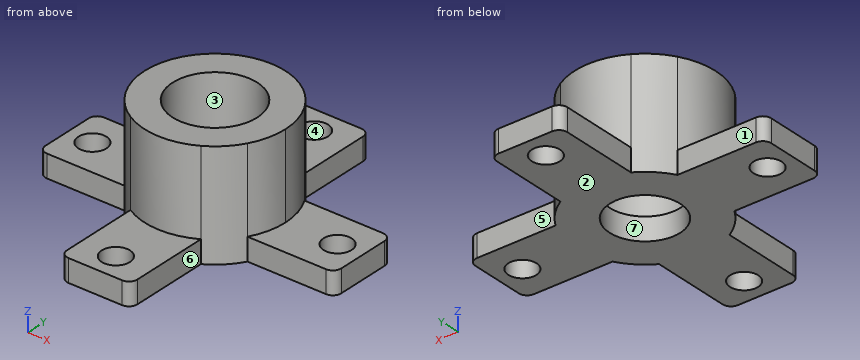
from build123d import *

# Parameters (mm, degrees)
F0_R     = 1
F0_W     = 5
F0_H     = 5
F1_DEPTH = 1.6
F2_R     = 3
F3_DEPTH = 6
F4_DEPTH = 1.6
F5_R     = 2.5
F6_DEPTH = 1.6


with BuildPart() as f1:
    # F0 (on Top) → F1 (new body)
    with BuildSketch(Plane.XY):
        with BuildLine():
            ThreePointArc((10.5, 1.9), (10.3242640687, 2.3242640687), (9.9, 2.5))
            Line((9.9, 2.5), (2.5, 2.5))
            Line((2.5, 2.5), (2.5, -2.5))
            Line((2.5, -2.5), (9.9, -2.5))
            ThreePointArc((9.9, -2.5), (10.3242640687, -2.3242640687), (10.5, -1.9))
            Line((10.5, -1.9), (10.5, 1.9))
        make_face()
        with Locations((8.7, 0)):
            Circle(F0_R, mode=Mode.SUBTRACT)
        Rectangle(F0_W, F0_H)
        with BuildLine():
            Line((-2.5, 2.5), (2.5, 2.5))
            Line((2.5, 2.5), (2.5, 9.9))
            ThreePointArc((2.5, 9.9), (2.3242640687, 10.3242640687), (1.9, 10.5))
            Line((1.9, 10.5), (-1.9, 10.5))
            ThreePointArc((-1.9, 10.5), (-2.3242640687, 10.3242640687), (-2.5, 9.9))
            Line((-2.5, 9.9), (-2.5, 2.5))
        make_face()
        with Locations((0, 8.7)):
            Circle(F0_R, mode=Mode.SUBTRACT)
        with BuildLine():
            Line((-2.5, -2.5), (-2.5, 2.5))
            Line((-2.5, 2.5), (-9.9, 2.5))
            ThreePointArc((-9.9, 2.5), (-10.3242640687, 2.3242640687), (-10.5, 1.9))
            Line((-10.5, 1.9), (-10.5, -1.9))
            ThreePointArc((-10.5, -1.9), (-10.3242640687, -2.3242640687), (-9.9, -2.5))
            Line((-9.9, -2.5), (-2.5, -2.5))
        make_face()
        with Locations((-8.7, 0)):
            Circle(F0_R, mode=Mode.SUBTRACT)
        with BuildLine():
            Line((2.5, -9.9), (2.5, -2.5))
            Line((2.5, -2.5), (-2.5, -2.5))
            Line((-2.5, -2.5), (-2.5, -9.9))
            ThreePointArc((-2.5, -9.9), (-2.3242640687, -10.3242640687), (-1.9, -10.5))
            Line((-1.9, -10.5), (1.9, -10.5))
            ThreePointArc((1.9, -10.5), (2.3242640687, -10.3242640687), (2.5, -9.9))
        make_face()
        with Locations((0, -8.7)):
            Circle(F0_R, mode=Mode.SUBTRACT)
    extrude(amount=F1_DEPTH)

    # F2 (on face) → F3 (join)
    with BuildSketch(Plane.XY.offset(1.6)):
        with BuildLine():
            ThreePointArc((4.3301270189, -2.5), (4.8296291314, -1.2940952255), (5, 0))
            ThreePointArc((5, 0), (4.8296291314, 1.2940952255), (4.3301270189, 2.5))
            Line((4.3301270189, 2.5), (2.5, 2.5))
            Line((2.5, 2.5), (2.5, 4.3301270189))
            ThreePointArc((2.5, 4.3301270189), (0, 5), (-2.5, 4.3301270189))
            Line((-2.5, 4.3301270189), (-2.5, 2.5))
            Line((-2.5, 2.5), (-4.3301270189, 2.5))
            ThreePointArc((-4.3301270189, 2.5), (-5, 0), (-4.3301270189, -2.5))
            Line((-4.3301270189, -2.5), (-2.5, -2.5))
            Line((-2.5, -2.5), (-2.5, -4.3301270189))
            ThreePointArc((-2.5, -4.3301270189), (0, -5), (2.5, -4.3301270189))
            Line((2.5, -4.3301270189), (2.5, -2.5))
            Line((2.5, -2.5), (4.3301270189, -2.5))
        make_face()
        Circle(F2_R, mode=Mode.SUBTRACT)
        with BuildLine():
            ThreePointArc((-4.3301270189, -2.5), (-3.5355339059, -3.5355339059), (-2.5, -4.3301270189))
            Line((-2.5, -4.3301270189), (-2.5, -2.5))
            Line((-2.5, -2.5), (-4.3301270189, -2.5))
        make_face()
        with BuildLine():
            ThreePointArc((2.5, -4.3301270189), (3.5355339059, -3.5355339059), (4.3301270189, -2.5))
            Line((4.3301270189, -2.5), (2.5, -2.5))
            Line((2.5, -2.5), (2.5, -4.3301270189))
        make_face()
        with BuildLine():
            Line((2.5, 2.5), (4.3301270189, 2.5))
            ThreePointArc((4.3301270189, 2.5), (3.5355339059, 3.5355339059), (2.5, 4.3301270189))
            Line((2.5, 4.3301270189), (2.5, 2.5))
        make_face()
        with BuildLine():
            Line((-2.5, 2.5), (-2.5, 4.3301270189))
            ThreePointArc((-2.5, 4.3301270189), (-3.5355339059, 3.5355339059), (-4.3301270189, 2.5))
            Line((-4.3301270189, 2.5), (-2.5, 2.5))
        make_face()
    extrude(amount=F3_DEPTH)

    # F4 (add, through all): faces of the model
    f4_faces = [f1.faces().sort_by_distance(p)[0] for p in [
        (-3.1629509292, 3.1629509292, 1.6),
        (3.1629509292, 3.1629509292, 1.6),
        (-3.1629509292, -3.1629509292, 1.6),
        (3.1629509292, -3.1629509292, 1.6),
    ]]
    extrude(f4_faces, amount=F4_DEPTH)

    # F5 (on face) → F6 (cut, through all)
    with BuildSketch(Plane.XY.offset(1.6)):
        Circle(F5_R)
    extrude(amount=-F6_DEPTH, mode=Mode.SUBTRACT)


solid = f1.part
Design review of the part built by this model. Coordinates are the model's own, in mm. Face numbers are marked on the shaded views. A direction names the side the tool comes from. Round coordinates to 2 decimals unless told otherwise and drop trailing zeros. Write each loop counter-clockwise with the first axis right and the second up, starting at its lowest first coordinate (ties: lowest second). Pieces come first, ordered by that corner, then holes. Notation, with made-up numbers: M 83,85.25 L 137,85.25 A17 ccw 137,105.25 Z; hole C -9,54 d11. An arc over 180 degrees is marked long. One line per item, written item: value. Start each with the question number.
1. Take a section at D-D on x = 5.5. State the section outline as (y, z) points, then the cut area to 3 significant figures.
2. Take a section at A-A on x = 0. State the section outline as (y, z) points, then the cut area to 3 significant figures.
3. Take a section at C-C on x = 8.7. State the section outline as (y, z) points, then the cut area to 3 significant figures.
4. Draft analysis for pull direction X (two halves, no side actions). For the marked faces 4, 5, 6 and 7, state which applies: pulls with the +X half, pulls with the -X half, needs draft (parallel to the pull), parting line crosses it, or undercut.
5. Clearance check with flat-ended pins moving along their axes: P1, Ø0.8, axis at y = -6.5, z = 0.5, coming from the +X side; P2, Ø2.5, axis at x = 0, y = -8.7, coming from the +Z side; P3, Ø1.3, axis at x = -7, z = 1, coming from the -Y side. State where each tip first meets the part, or that it passes through.
6. For the marked faces 1, 2 and 3, list the 3-axis set-ups (+Z, -Z, +X, -X, +Y, -Y) from which the entire face can be reached by the end or side of a thin tool; tool diameter is ignored.
7. Take a section at B-B on z = 2. State the section outline as (x, y) points.
8. To check wall thickness, follow probe 1 along Y at (x, z) = (0, 0.9); probe 2 along Y at (x, z) = (0, 3.45); probe 3 along Y at (x, z) = (-8.7, 1.15). State the ranges of each line that lie inside material, in increasing order. Write a range as from..to.
Computed:
1. outline: M -2.5,0 L 2.5,0 L 2.5,1.6 L -2.5,1.6 Z
1. area: 8.00 mm²
2. outline: M -10.5,0 L -9.7,0 L -9.7,1.6 L -10.5,1.6 Z; M -7.7,0 L -2.5,0 L -2.5,1.6 L -3,1.6 L -3,7.6 L -5,7.6 L -5,1.6 L -7.7,1.6 Z; M 2.5,0 L 7.7,0 L 7.7,1.6 L 5,1.6 L 5,7.6 L 3,7.6 L 3,1.6 L 2.5,1.6 Z; M 9.7,0 L 10.5,0 L 10.5,1.6 L 9.7,1.6 Z
2. area: 43.2 mm²
3. outline: M -2.5,0 L -1,0 L -1,1.6 L -2.5,1.6 Z; M 1,0 L 2.5,0 L 2.5,1.6 L 1,1.6 Z
3. area: 4.80 mm²
4. face 4: undercut
4. face 5: needs draft
4. face 6: pulls with the +X half
4. face 7: undercut
5. P1: stops at x = 2.5
5. P2: stops at z = 1.6
5. P3: stops at y = -2.5
6. face 1: +Z, -Z, -X, +Y
6. face 2: -Z, +X, -X, +Y, -Y
6. face 3: +Z
7. outline: C 0,0 d10; hole C 0,0 d6
8. probe 1: y = -10.5..-9.7, -7.7..-2.5, 2.5..7.7, 9.7..10.5
8. probe 2: y = -5..-3, 3..5
8. probe 3: y = -2.5..-1, 1..2.5
